Work out the finished part from the listing and answer in its coordinate system (mm). A direction names the side the tool comes from. Round coordinates to 2 decimals unless told otherwise and drop trailing zeros. Loops run counter-clockwise (first coordinate to the right, second up) from the corner with the lowest first, then second, coordinate; pieces in that order, holes last.
```python
from build123d import *

# Parameters (mm, degrees)
BOSS_EXTRUDE1_DEPTH         = 3.175
SKETCH2_W                   = 2.75
SKETCH2_H                   = 2.5
SKETCH2_H_2                 = 4
SKETCH2_W_2                 = 1.125
SKETCH2_H_3                 = 7.5
CUT_EXTRUDE1_DEPTH          = 174.529048361
CIRPATTERN1_COUNT           = 4
F_3_0_3_DIAMETER_HOLE1_D    = 3
F_3_8_CLEARANCE_HOLE1_D     = 10.31748
F_3_8_CLEARANCE_HOLE1_DEPTH = 6.35
F_4_CLEARANCE_HOLE1_D       = 3.4544


with BuildPart() as part:
    # Sketch1 → Boss-Extrude1 (new, symmetric)
    with BuildSketch(Plane(origin=(0, 0, 0), x_dir=(1, 0, 0), z_dir=(0, 1, 0))):
        with BuildLine():
            ThreePointArc((88.101844639, -45.675437768), (-70.171862751, 70.171862751), (45.675437768, -88.101844639))
            Line((45.675437768, -88.101844639), (80.256619665, -122.683026536))
            Line((80.256619665, -122.683026536), (122.683026536, -80.256619665))
            Line((122.683026536, -80.256619665), (88.101844639, -45.675437768))
        make_face()
        with BuildLine():
            Line((-83.903460262, -7.5), (-7.5, -7.5))
            Line((-7.5, -7.5), (-7.5, -83.903460262))
            ThreePointArc((-7.5, -83.903460262), (-59.565261034, -59.565261034), (-83.903460262, -7.5))
        make_face(mode=Mode.SUBTRACT)
        with BuildLine():
            ThreePointArc((83.903460262, -7.5), (59.565261034, -59.565261034), (7.5, -83.903460262))
            Line((7.5, -83.903460262), (7.5, -7.5))
            Line((7.5, -7.5), (83.903460262, -7.5))
        make_face(mode=Mode.SUBTRACT)
        with BuildLine():
            ThreePointArc((-83.903460262, 7.5), (-59.565261034, 59.565261034), (-7.5, 83.903460262))
            Line((-7.5, 83.903460262), (-7.5, 7.5))
            Line((-7.5, 7.5), (-83.903460262, 7.5))
        make_face(mode=Mode.SUBTRACT)
        with BuildLine():
            ThreePointArc((7.5, 83.903460262), (59.565261034, 59.565261034), (83.903460262, 7.5))
            Line((83.903460262, 7.5), (7.5, 7.5))
            Line((7.5, 7.5), (7.5, 83.903460262))
        make_face(mode=Mode.SUBTRACT)
    extrude(amount=BOSS_EXTRUDE1_DEPTH, both=True)

    # Sketch2 → Cut-Extrude1 (cut, symmetric)
    with BuildSketch(Plane(origin=(0, 0, 0), x_dir=(1, 0, 0), z_dir=(0, 1, 0))):
        with Locations((0, 86.488)):
            Rectangle(SKETCH2_W, SKETCH2_H)
        with Locations((0, 89.738)):
            Rectangle(SKETCH2_W, SKETCH2_H_2)
        with Locations((1.9375, 89.738)):
            Rectangle(SKETCH2_W_2, SKETCH2_H_2)
        with Locations((0, 95.488)):
            Rectangle(SKETCH2_W, SKETCH2_H_3)
        with Locations((-1.9375, 89.738)):
            Rectangle(SKETCH2_W_2, SKETCH2_H_2)
    cut_extrude1 = extrude(amount=CUT_EXTRUDE1_DEPTH, both=True, mode=Mode.SUBTRACT)

    # CirPattern1: Cut-Extrude1 ×4 about axis
    cirpattern1_axis = Axis((0, 0, 0), (0, 1, 0))
    for i in range(1, CIRPATTERN1_COUNT):
        add(cut_extrude1.rotate(cirpattern1_axis, i * 360 / CIRPATTERN1_COUNT), mode=Mode.SUBTRACT)

    # Ø3.0 (3) Diameter Hole1 (through all)
    with Locations(Plane(origin=(0, 3.175, 0), x_dir=(1, 0, 0), z_dir=(0, 1, 0))):
        with Locations((-64.868561892, -64.868561892), (0, 0), (-64.868561892, 64.868561892), (64.868561892, 64.868561892), (64.868561892, -64.868561892)):
            Hole(F_3_0_3_DIAMETER_HOLE1_D / 2)

    # 3/8 Clearance Hole1
    with Locations(Plane(origin=(0, 3.175, 0), x_dir=(1, 0, 0), z_dir=(0, 1, 0))):
        with Locations((0, 0)):
            Hole(F_3_8_CLEARANCE_HOLE1_D / 2, depth=F_3_8_CLEARANCE_HOLE1_DEPTH)

    # #4 Clearance Hole1 (through all)
    with Locations(Plane(origin=(0, 3.175, 0), x_dir=(1, 0, 0), z_dir=(0, 1, 0))):
        with Locations((15.88, -3.94), (15.88, 3.94)):
            Hole(F_4_CLEARANCE_HOLE1_D / 2)


solid = part.part
```
1. Given pin 1 (2 mm diameter, centred on x = 71.5, y = 1.5, fed in from +Z); pin 2 (5 mm diameter, centred on x = 64.87, z = 64.87, fed in from +Y) (3 decimals); pin 3 (1.4 mm diameter, centred on y = 0, z = -0.5, fed in from -X); pin 4 (2 mm diameter, centred on x = -90, y = 1, fed in from -Z), each flat-ended and moving along its own axis, determine where each tip first touches the part or whether it passes through.
Answer key:
pin 1: stops at z = 114.93
pin 2: stops at y = 3.175
pin 3: stops at x = -85.24
pin 4: stops at z = -43.9
2. Determine the mould class of faces 1 (the face through (-95, 0, -1.375)), 2 (the face through (1.375, 0, -95)), 3 (the face through (62.724, 0.044, 105.15)), 4 (the face through (60.143, 0.044, 58.982)) for opening direction Z: +Z half, -Z half, draft (parallel to the pull), parting line (faces both ways), or undercut.
Answer key:
face 1: undercut
face 2: draft
face 3: +Z half
face 4: undercut
3. Which of the six approach directions +Z, -Z, +X, -X, +Y, -Y give full straight-line access (tool end or side, diameter ignored) to faces 5 (the face through (-1.375, 0, -96)), 6 (the face through (23.861, 0.044, 96.327)), 7 (the face through (-96, 0, 1.375)), 8 (the face through (95, 0, 1.375)), 9 (the face through (-46, 0, 7.5))?
Answer key:
face 5: -Z, +Y, -Y
face 6: +Z, +Y, -Y
face 7: -X, +Y, -Y
face 8: +X, +Y, -Y
face 9: +Y, -Y
4. Find section B-B (z = -26.5). Write down the section's boundary in (x, y) (3 decimals), then the cut area to 3 significant figures.
Answer key:
outline: (-95.634, -3.175) - (-79.961, -3.175) - (-79.961, 3.175) - (-95.634, 3.175) - close; (-7.5, -3.175) - (7.5, -3.175) - (7.5, 3.175) - (-7.5, 3.175) - close; (79.961, -3.175) - (95.634, -3.175) - (95.634, 3.175) - (79.961, 3.175) - close
area: 294 mm2
5. Consider probe 1 along Z at (x, y) = (58, 0.5); probe 2 along Z at (x, y) = (15.88, 1); probe 3 along X at (y, z) = (-1.5, -21). Determine where each line is inside the solid, lowest interval first.
Answer key:
probe 1: z = -80.52 to -61.09, -7.5 to 7.5, 61.09 to 100.43
probe 2: z = -97.96 to -82.73, -7.5 to -5.67, -2.21 to 2.21, 5.67 to 7.5, 82.73 to 97.96
probe 3: x = -96.99 to -81.58, -7.5 to 7.5, 81.58 to 96.99
6. Find section A-A (x = 31). Write down the section's boundary in (y, z) (1 decimal).
Answer key:
outline: (-3.2, -94.3) - (3.2, -94.3) - (3.2, -78.3) - (-3.2, -78.3) - close; (-3.2, -7.5) - (3.2, -7.5) - (3.2, 7.5) - (-3.2, 7.5) - close; (-3.2, 78.3) - (3.2, 78.3) - (3.2, 94.3) - (-3.2, 94.3) - close
7. Find section C-C (y = 1). Give the number of separate pieces and of enclosed holes in the cut face, then the cut area to 3 significant figures.
Answer key:
separate pieces: 1
enclosed holes: 11
area: 15,900 mm2
